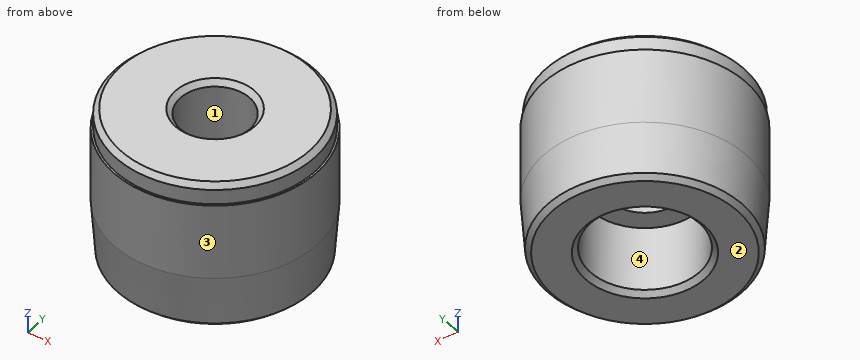
```python
from build123d import *


# Not quite as in the source:
# - a fillet or chamfer that OpenCascade refuses, or shapes differently, is made with other operations: its cross-section is extruded or revolved along the edge and cut away or added


with BuildPart() as f1:
    # F0 (on Front) → F1 (revolve)
    with BuildSketch(Plane.XZ):
        Polygon((-3.5, -0.575), (-3.5, 7.575), (-10, 7.575), (-10, 5.575), (-10.2, 5.575), (-10.2, -2.075), (-9.8, -7.575), (-5.5, -7.575), (-5.5, -0.575), align=None)
    revolve(axis=Axis((0, 0, 0.3696661443), (0, 0, -1)))

    # F2: chamfer of 0.5 on 4 edges, made by hand

    # F2_s1 → F2_t2 (revolve, cut)
    with BuildSketch(Plane.XZ):
        Polygon((-6, -7.575), (-5.5, -7.075), (-5.5, -7.575), align=None)
    revolve(axis=Axis((0, 0, -7.575), (0, 0, -1)), mode=Mode.SUBTRACT)

    # F2_s3 → F2_t4 (revolve, cut)
    with BuildSketch(Plane.XZ):
        Polygon((-9.8337259747, -7.1112678479), (-9.3350430662, -7.575), (-9.8, -7.575), align=None)
    revolve(axis=Axis((0, 0, -7.575), (0, 0, -1)), mode=Mode.SUBTRACT)

    # F2_s5 → F2_t6 (revolve, cut)
    with BuildSketch(Plane.XZ):
        Polygon((-9.5, 7.575), (-10, 7.075), (-10, 7.575), align=None)
    revolve(axis=Axis((0, 0, 7.575), (0, 0, -1)), mode=Mode.SUBTRACT)

    # F2_s7 → F2_t8 (revolve, cut)
    with BuildSketch(Plane.XZ):
        Polygon((-3.5, 7.075), (-4, 7.575), (-3.5, 7.575), align=None)
    revolve(axis=Axis((0, 0, 7.575), (0, 0, -1)), mode=Mode.SUBTRACT)


solid = f1.part
```
Could you check a few things on this model? Use its own coordinates, in mm. Face numbers are marked on the shaded views. Coordinates: 2 decimals unless noted, no trailing zeros. Loops run counter-clockwise (first coordinate to the right, second up) from the corner with the lowest first, then second, coordinate; pieces in that order, holes last. Notation, with made-up numbers: M 42,85.25 L 61,85.25 A18 cw 61,118.25 Z; hole C -7.75,58.5 d3. An arc over 180 degrees is marked long. Put each result on its own line as item: value. Start each with the question number.
(1) Will these pins go through, and if not, where does the flat tip stop? P1, Ø3.5, axis at x = -2.5, y = 0, coming from the -Z side (3 decimals); P2, Ø4, axis at y = 7, z = 2.5, coming from the -X side; P3, Ø3, axis at x = -4, y = -2, coming from the -Z side.
(2) Thinking about a two-plate mould opening in X: for the marked faces 1, 2, 3 and 4, which applies, pulls with the +X half, pulls with the -X half, needs draft (parallel to the pull), parting line crosses it, or undercut?
(3) Suppose I cut it at C-C on z = 6.5. Please give me the cut outline in (x, y), then the cut area to 3 significant figures.
(4) Suppose I cut it at D-D on z = 3.25. Please give me the cut outline in (x, y).
(5) I need wall thicknesses on line 1 (Y direction, x = 0, z = 3.5); line 2 (Y direction, x = 0, z = -2); line 3 (Z direction, x = 4, y = 2.5) (3 decimals). Which ranges of each line are inside material? Lowest first, please. Write a range as from..to.
(6) Suppose I cut it at A-A on y = 0. Please give me the cut outline in (x, z) (3 decimals), then the cut area to 3 significant figures.
Solutions:
1. P1: stops at z = -0.575
1. P2: stops at x = -8.89
1. P3: stops at z = -7.55
2. face 1: undercut
2. face 2: needs draft
2. face 3: parting line crosses it
2. face 4: undercut
3. outline: C 0,0 d20; hole C 0,0 d7
3. area: 276 mm2
4. outline: C 0,0 d20.4; hole C 0,0 d7
5. line 1: y = -10.2..-3.5, 3.5..10.2
5. line 2: y = -10.2..-5.5, 5.5..10.2
5. line 3: z = -0.575..7.575
6. outline: M -10.2,-2.075 L -9.834,-7.111 L -9.335,-7.575 L -6,-7.575 L -5.5,-7.075 L -5.5,-0.575 L -3.5,-0.575 L -3.5,7.075 L -4,7.575 L -9.5,7.575 L -10,7.075 L -10,5.575 L -10.2,5.575 Z; M 3.5,-0.575 L 5.5,-0.575 L 5.5,-7.075 L 6,-7.575 L 9.335,-7.575 L 9.834,-7.111 L 10.2,-2.075 L 10.2,5.575 L 10,5.575 L 10,7.075 L 9.5,7.575 L 4,7.575 L 3.5,7.075 Z
6. area: 171 mm2
